Verification items for the finished model (mm, model axes). A direction names the side the tool comes from. Round coordinates to 2 decimals unless told otherwise and drop trailing zeros. Order: outer loops, then holes, each group sorted by start corner. A loop starts at its lowest first (then second) coordinate and runs counter-clockwise, first axis right, second up. Notation, with made-up numbers: (-28, 18) -> (27, 18) arc R14 ccw to (27, 38) -> close; hole circle Ø2 at (70.25, -27.5). An arc over 180 degrees is marked (long way). Answer in a Markdown table with one row per item. Add a question column.
```python
from build123d import *

# Parameters (mm, degrees)
F0_R     = 37.956289
F1_DEPTH = 127.45938
F2_W     = 33.085958
F2_H     = 31.139728
F3_DEPTH = 63.29228
F5_D     = 6.35


with BuildPart() as f1:
    # F0 (on Front) → F1 (new body)
    with BuildSketch(Plane.XZ):
        Circle(F0_R)
    extrude(amount=F1_DEPTH)

    # F2 (on Top) → F3 (join)
    with BuildSketch(Plane.XY):
        with Locations((-30.166611, -51.782193)):
            Rectangle(F2_W, F2_H)
    extrude(amount=F3_DEPTH)

    # F5 (through all)
    with Locations(Plane.XY.offset(63.29228)):
        with Locations((-30.711466, -51.782193)):
            Hole(F5_D / 2)


solid = f1.part
```
1) Cross-section at C-C, the plane x = 0. Record the boundary of the cut face in (y, z), and give its area (3 significant figures).
2) Draft check along Y on faces 1 (the face through (-1, -127.459, 1)), 2 (the face through (-27.54, -51.64, 17.96)), 3 (the face through (-42, -52, 0)). Enter one of: +Y half, -Y half, draft (parallel to the pull), parting line (faces both ways), or undercut.
3) Cross-section at B-B, the plane y = -71. Record the boundary of the cut face in (x, z), and give its area (3 significant figures).
4) Depth check by flat-ended pin: P1, Ø1, axis at x = 24, y = -83, coming from the -Z side; P2, Ø12, axis at x = -21, y = -71, coming from the -Z side; P3, Ø12, axis at y = -69.5, z = -18, coming from the -X side. Enter the tip coordinate at first touch or a pass-through.
5) Thickness scan on L1, parallel to Y at x = -39, z = 20; L2, parallel to X at y = -59.5, z = -1; L3, parallel to X at y = -49, z = 4. Record the ranges inside material, lowest first. Write a range as [from, to].
6) Tool access check on faces 4 (the face through (-34, -36.212, 38)), 5 (the face through (-46.71, -52, 31)), 6 (the face through (-34, -67.352, 38)). Record the directions out of +Z, -Z, +X, -X, +Y, -Y that give a thin tool (end or side, any length) a straight path to the whole face; none if there is none.
7) Cross-section at D-D, the plane z = -11.5. Record the boundary of the cut face in (x, y) (3 decimals), and give its area (3 significant figures).
8) Cross-section at A-A, the plane z = 7.5. Record the boundary of the cut face in (x, y) (3 decimals).
Results below:
| question | item | result |
|---|---|---|
| 1 | outline | (-127.46, -37.96) -> (0, -37.96) -> (0, 37.96) -> (-127.46, 37.96) -> close |
| 1 | area | 9,680 mm² |
| 2 | face 1 | -Y half |
| 2 | face 2 | undercut |
| 2 | face 3 | draft |
| 3 | outline | circle Ø75.91 at (0, 0) |
| 3 | area | 4,530 mm² |
| 4 | P1 | z = -29.81 |
| 4 | P2 | z = -34.87 |
| 4 | P3 | x = -36.01 |
| 5 | L1 | [-67.35, -36.21] |
| 5 | L2 | [-37.94, 37.94] |
| 5 | L3 | [-46.71, -32.24], [-29.18, 37.74] |
| 6 | face 4 | +Z, -X, +Y |
| 6 | face 5 | +Z, -Z, -X, +Y, -Y |
| 6 | face 6 | +Z, -X, -Y |
| 7 | outline | (-36.172, -127.459) -> (36.172, -127.459) -> (36.172, 0) -> (-36.172, 0) -> close; hole circle Ø6.35 at (-30.711, -51.782) |
| 7 | area | 9,190 mm² |
| 8 | outline | (-46.71, -67.352) -> (-37.208, -67.352) -> (-37.208, -127.459) -> (37.208, -127.459) -> (37.208, 0) -> (-37.208, 0) -> (-37.208, -36.212) -> (-46.71, -36.212) -> close; hole circle Ø6.35 at (-30.711, -51.782) |
